```python
from build123d import *

# Parameters (mm, degrees)
BOSS_EXTRUDE1_DEPTH     = 5
CUT_EXTRUDE2_START      = -75.1
SKETCH3_W               = 20
SKETCH3_H               = 5
CUT_EXTRUDE2_DEPTH      = 14.477720111
CUT_EXTRUDE3_DEPTH      = 89.577720111
CUT_EXTRUDE3_DEPTH_BACK = 89.577720111
SKETCH4_R               = 2.5


with BuildPart() as part:
    # Sketch1 → Boss-Extrude1 (new, symmetric)
    with BuildSketch(Plane(origin=(0, 0, 0), x_dir=(1, 0, 0), z_dir=(0, 1, 0))):
        Polygon((-24.706854249, 39.55), (24.706854249, 39.55), (39.55, 24.706854249), (39.55, -24.706854249), (24.706854249, -39.55), (-24.706854249, -39.55), (-39.55, -24.706854249), (-39.55, 24.706854249), align=None)
        Polygon((-35.55, 23.05), (-23.05, 35.55), (23.05, 35.55), (35.55, 23.05), (35.55, -23.05), (23.05, -35.55), (-23.05, -35.55), (-35.55, -23.05), align=None, mode=Mode.SUBTRACT)
    extrude(amount=BOSS_EXTRUDE1_DEPTH, both=True)

    # Sketch3 → Cut-Extrude2 (cut, through all)
    with BuildSketch(Plane(origin=(39.55, 0, 0), x_dir=(0, 0, -1), z_dir=(1, 0, 0)).offset(CUT_EXTRUDE2_START)):
        Rectangle(SKETCH3_W, SKETCH3_H)
    extrude(amount=-CUT_EXTRUDE2_DEPTH, mode=Mode.SUBTRACT)

    # Sketch4 → Cut-Extrude3 (cut, two sides: drawn at the far end of the back side and taken through both)
    with BuildSketch(Plane(origin=(0, 0, -39.55), x_dir=(-1, 0, 0), z_dir=(0, 0, -1)).offset(-CUT_EXTRUDE3_DEPTH_BACK)):
        with Locations(Location((0, 0, 0), (0, 0, 180))):
            Circle(SKETCH4_R)
    extrude(amount=CUT_EXTRUDE3_DEPTH + CUT_EXTRUDE3_DEPTH_BACK, mode=Mode.SUBTRACT)


solid = part.part
```
CAD build for the part. Positions are in the model's coordinates, mm. A direction names the side the tool comes from. Round coordinates to 2 decimals unless told otherwise and drop trailing zeros. Write each loop counter-clockwise with the first axis right and the second up, starting at its lowest first coordinate (ties: lowest second). Pieces come first, ordered by that corner, then holes. Notation, with made-up numbers: (63.5, 83.25) -> (105.5, 83.25) arc R13 ccw to (105.5, 105.25) -> close; hole circle Ø1 at (-38.75, -22.5). An arc over 180 degrees is marked (long way). Answer in a Markdown table with one row per item. Add a question column.
Item 1: Saw through at D-D, the plane x = 26. Write the cut outline in (y, z).
Item 2: Which spindle directions (+Z, -Z, +X, -X, +Y, -Y) get a long thin tool onto all of the face, cutting with end or side? Do faces 1 (the face through (0, 3, 39.55)), 2 (the face through (-38, 2.5, 0)), 3 (the face through (0, 3, -35.55)). Say none if no direction does.
Item 3: Drill centre lines: line 1 (Y direction, x = 0, z = 38.4); line 2 (X direction, y = 0, z = 19.5). Where is each one in solid material? Low to high. Write a range as from..to.
Item 4: Drop flat-ended pins along their axis: pin 1 Ø4.5 at (x, y) = (-38.5, -1) entering from -Z; pin 2 Ø1.5 at (y, z) = (-2.5, -30.5) entering from +X; pin 3 Ø1.5 at (y, z) = (4, 28) entering from -X. Give the stop position or say it passes through.
Item 5: Mould opens along X. For faces 4 (the face through (38, 5, 0)), 5 (the face through (-32.232, 0.07, -32.025)), 6 (the face through (29.2, 0.1, -29.4)), 7 (the face through (29.4, 0.1, 29.2)) say: pulls with the +X half, pulls with the -X half, needs draft (parallel to the pull), parting line crosses it, or undercut.
Item 6: Saw through at B-B, the plane z = -14.5. Write the cut outline in (x, y), then the cut area to 3 significant figures.
Item 7: Saw through at C-C, the plane z = 1. Write the cut outline in (x, y).
Item 8: Saw through at A-A, the plane x = 0. Write the cut outline in (y, z).
Findings below:
| question | item | result |
|---|---|---|
| 1 | outline | (-5, -38.26) -> (5, -38.26) -> (5, -32.6) -> (-5, -32.6) -> close; (-5, 32.6) -> (5, 32.6) -> (5, 38.26) -> (-5, 38.26) -> close |
| 2 | face 1 | +Z, +X, -X, +Y, -Y |
| 2 | face 2 | -X |
| 2 | face 3 | +Y, -Y |
| 3 | line 1 | y = -5..-2.5, 2.5..5 |
| 3 | line 2 | x = -39.55..-35.55, 35.55..39.55 |
| 4 | pin 1 | stops at z = -28.01 |
| 4 | pin 2 | stops at x = 34.51 |
| 4 | pin 3 | stops at x = -37.01 |
| 5 | face 4 | needs draft |
| 5 | face 5 | pulls with the -X half |
| 5 | face 6 | undercut |
| 5 | face 7 | undercut |
| 6 | outline | (-39.55, -5) -> (-35.55, -5) -> (-35.55, 5) -> (-39.55, 5) -> close; (35.55, -5) -> (39.55, -5) -> (39.55, 5) -> (35.55, 5) -> close |
| 6 | area | 80.0 mm^2 |
| 7 | outline | (-39.55, -5) -> (-35.55, -5) -> (-35.55, -2.5) -> (-39.55, -2.5) -> close; (-39.55, 2.5) -> (-35.55, 2.5) -> (-35.55, 5) -> (-39.55, 5) -> close; (35.55, -5) -> (39.55, -5) -> (39.55, 5) -> (35.55, 5) -> close |
| 8 | outline | (-5, -39.55) -> (-2.5, -39.55) -> (-2.5, -35.55) -> (-5, -35.55) -> close; (-5, 35.55) -> (-2.5, 35.55) -> (-2.5, 39.55) -> (-5, 39.55) -> close; (2.5, -39.55) -> (5, -39.55) -> (5, -35.55) -> (2.5, -35.55) -> close; (2.5, 35.55) -> (5, 35.55) -> (5, 39.55) -> (2.5, 39.55) -> close |
